Geometry: final body of the model. Coordinates: model frame, mm. Face numbers are marked on the shaded views. A direction names the side the tool comes from. Round coordinates to 2 decimals unless told otherwise and drop trailing zeros. Write each loop counter-clockwise with the first axis right and the second up, starting at its lowest first coordinate (ties: lowest second). Pieces come first, ordered by that corner, then holes. Notation, with made-up numbers: (38.5, 17.5) -> (92.5, 17.5) arc R4 cw to (92.5, 24.5) -> close; hole circle Ø2 at (63.25, 66). An arc over 180 degrees is marked (long way). Use one line per item in the form item = value. Start each with the question number.
1. Cut plane D-D, the plane y = -18.5. Return the cut outline in (x, z).
2. Reachability of the marked faces 1, 2, 3 and 4 from +Z, -Z, +X, -X, +Y, -Y: full face, straight path, thin tool, end or side. Return the list, or none.
3. Pin query (flat end, axial travel): pin 1 Ø8 at (x, y) = (40, -38.5) entering from -Z; pin 2 Ø14 at (x, y) = (26.5, -48) entering from +Z; pin 3 Ø2 at (x, z) = (-19, -16) entering from +Y. Return the tip coordinate at first contact, or that it passes through.
4. Line query: L1, parallel to Y at x = 77, z = -44; L2, parallel to Z at x = -79, y = -14; L3, parallel to Z at x = -6.5, y = -37. Output: solid intervals per line, ascending.
5. Cut plane C-C, the plane z = -22. Return the cut outline in (x, y).
6. Draft query along X for the marked faces 5, 6 and 7. Return one class per face: pulls with the +X half, pulls with the -X half, needs draft (parallel to the pull), parting line crosses it, or undercut.
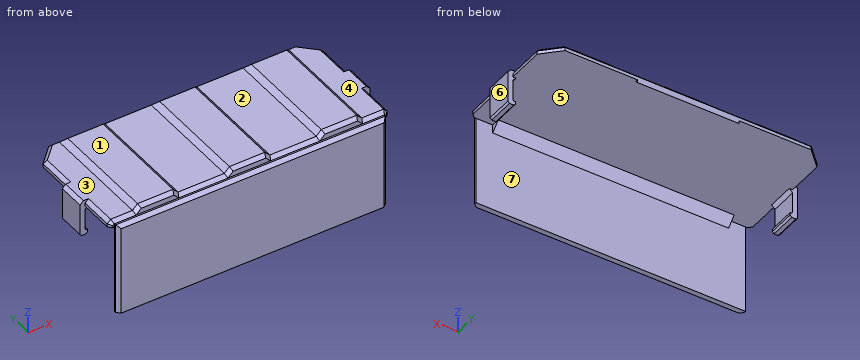
```python
from build123d import *

# Parameters (mm, degrees)
SKETCH1_W           = 166
SKETCH1_H           = 70
BOSS_EXTRUDE1_DEPTH = 4
CHAMFER1_SIZE       = 10
CHAMFER2_SIZE       = 2
BOSS_EXTRUDE2_DEPTH = 68
CHAMFER3_SIZE       = 3
SKETCH3_W           = 160
SKETCH3_H           = 55
BOSS_EXTRUDE3_DEPTH = 3
CHAMFER4_SIZE       = 2
BOSS_EXTRUDE4_DEPTH = 140
BOSS_EXTRUDE5_DEPTH = 16
CHAMFER5_SIZE       = 0.75
CHAMFER6_SIZE       = 2
CHAMFER7_SIZE       = 2
BOSS_EXTRUDE6_DEPTH = 30


with BuildPart() as part:
    # Sketch1 → Boss-Extrude1 (new body)
    with BuildSketch(Plane.XY):
        with Locations((0, -35)):
            Rectangle(SKETCH1_W, SKETCH1_H)
    extrude(amount=BOSS_EXTRUDE1_DEPTH)

    # Chamfer1
    chamfer1_edges = [part.edges().sort_by_distance(p)[0] for p in [
        (-83, 0, 2),
        (83, 0, 2),
    ]]
    chamfer(chamfer1_edges, length=CHAMFER1_SIZE)

    # Chamfer2
    chamfer2_edges = [part.edges().sort_by_distance(p)[0] for p in [
        (-83, -40, 4),
        (0, 0, 4),
        (78, -5, 4),
        (-78, -5, 4),
        (83, -40, 4),
    ]]
    chamfer(chamfer2_edges, length=CHAMFER2_SIZE)

    # Sketch2 → Boss-Extrude2 (add)
    with BuildSketch(Plane(origin=(0, -70, 0), x_dir=(-1, 0, 0), z_dir=(0, -1, 0))):
        Polygon((68, -4), (65, -7), (44, -7), (41, -4), align=None)
        Polygon((13.5, -4), (-13.5, -4), (-10.5, -7), (10.5, -7), align=None)
        Polygon((-41, -4), (-44, -7), (-65, -7), (-68, -4), align=None)
    extrude(amount=-BOSS_EXTRUDE2_DEPTH)

    # Chamfer3
    chamfer3_edges = [part.edges().sort_by_distance(p)[0] for p in [
        (54.5, -2, 7),
        (0, -2, 7),
        (-54.5, -2, 7),
    ]]
    chamfer(chamfer3_edges, length=CHAMFER3_SIZE - 0.0001)  # a hair under: the kernel refuses the full size

    # Sketch3 → Boss-Extrude3 (add)
    with BuildSketch(Plane(origin=(0, -70, 0), x_dir=(-1, 0, 0), z_dir=(0, -1, 0))):
        with Locations((0, 25.5)):
            Rectangle(SKETCH3_W, SKETCH3_H)
    extrude(amount=BOSS_EXTRUDE3_DEPTH)

    # Chamfer4
    chamfer4_edges = [part.edges().sort_by_distance(p)[0] for p in [
        (80, -73, -25.5),
        (0, -73, 2),
        (-80, -73, -25.5),
    ]]
    chamfer(chamfer4_edges, length=CHAMFER4_SIZE)

    # Sketch4 → Boss-Extrude4 (add)
    with BuildSketch(Plane.ZY.offset(70)):
        Polygon((0, -70), (0, -65), (-5, -70), align=None)
    extrude(amount=-BOSS_EXTRUDE4_DEPTH)

    # Sketch5 → Boss-Extrude5 (add)
    with BuildSketch(Plane(origin=(0, -48, 0), x_dir=(-1, 0, 0), z_dir=(0, -1, 0))):
        Polygon((-81, -4), (-83, -2), (-83, 15), (-81.5, 15), (-81.5, 16.5), (-82.5, 17.5), (-85, 17.5), (-86, 16.5), (-86, -2), (-84, -4), align=None)
        Polygon((81.5, 16.5), (82.5, 17.5), (85, 17.5), (86, 16.5), (86, -2), (84, -4), (81, -4), (83, -2), (83, 15), (81.5, 15), align=None)
    extrude(amount=-BOSS_EXTRUDE5_DEPTH)

    # Chamfer5
    chamfer5_edges = [part.edges().sort_by_distance(p)[0] for p in [
        (83, -40, -15),
        (-83, -40, -15),
    ]]
    chamfer(chamfer5_edges, length=CHAMFER5_SIZE)

    # Chamfer6
    chamfer6_edges = [part.edges().sort_by_distance(p)[0] for p in [
        (83, -40, 0),
        (-83, -40, 0),
    ]]
    chamfer(chamfer6_edges, length=CHAMFER6_SIZE)

    # Chamfer7
    chamfer7_edges = [part.edges().sort_by_distance(p)[0] for p in [
        (-74.5, -70, 4),
        (83, -70, 1),
        (-83, -70, 1),
        (-82, -70, 3),
        (82, -70, 3),
        (-27.25, -70, 4),
        (-42.5, -70, 5.5),
        (-54.5, -70, 7),
        (-66.5, -70, 5.5),
        (27.25, -70, 4),
        (-12, -70, 5.5),
        (12, -70, 5.5),
        (0, -70, 7),
        (74.5, -70, 4),
        (66.5, -70, 5.5),
        (54.5, -70, 7),
        (42.5, -70, 5.5),
    ]]
    chamfer(chamfer7_edges, length=CHAMFER7_SIZE - 0.0001)  # a hair under: the kernel refuses the full size

    # Sketch6 → Boss-Extrude6 (add, symmetric)
    with BuildSketch(Plane(origin=(0, 0, 0), x_dir=(0, 0, -1), z_dir=(1, 0, 0))):
        Polygon((0, -1.75), (1.75, 0), (0, 0), align=None)
    extrude(amount=BOSS_EXTRUDE6_DEPTH, both=True)


solid = part.part
```
Outcome:
q1.outline = (-83, 0) -> (83, 0) -> (83, 2) -> (81, 4) -> (68, 4) -> (65, 7) -> (44, 7) -> (41, 4) -> (13.5, 4) -> (10.5, 7) -> (-10.5, 7) -> (-13.5, 4) -> (-41, 4) -> (-44, 7) -> (-65, 7) -> (-68, 4) -> (-81, 4) -> (-83, 2) -> close
q2.face_1 = +Z, +X, -X, +Y, -Y
q2.face_2 = +Z, +Y, -Y
q2.face_3 = +Z, -X, +Y, -Y
q2.face_4 = +Z, +X, +Y, -Y
q3.pin_1 = 0
q3.pin_2 = 4
q3.pin_3 = -70
q4.L1 = -73 to -70
q4.L2 = 0 to 4
q4.L3 = 0 to 7
q5.outline = (-80, -71) -> (-78, -73) -> (78, -73) -> (80, -71) -> (80, -70) -> (-80, -70) -> close
q6.face_5 = undercut
q6.face_6 = pulls with the +X half
q6.face_7 = needs draft
